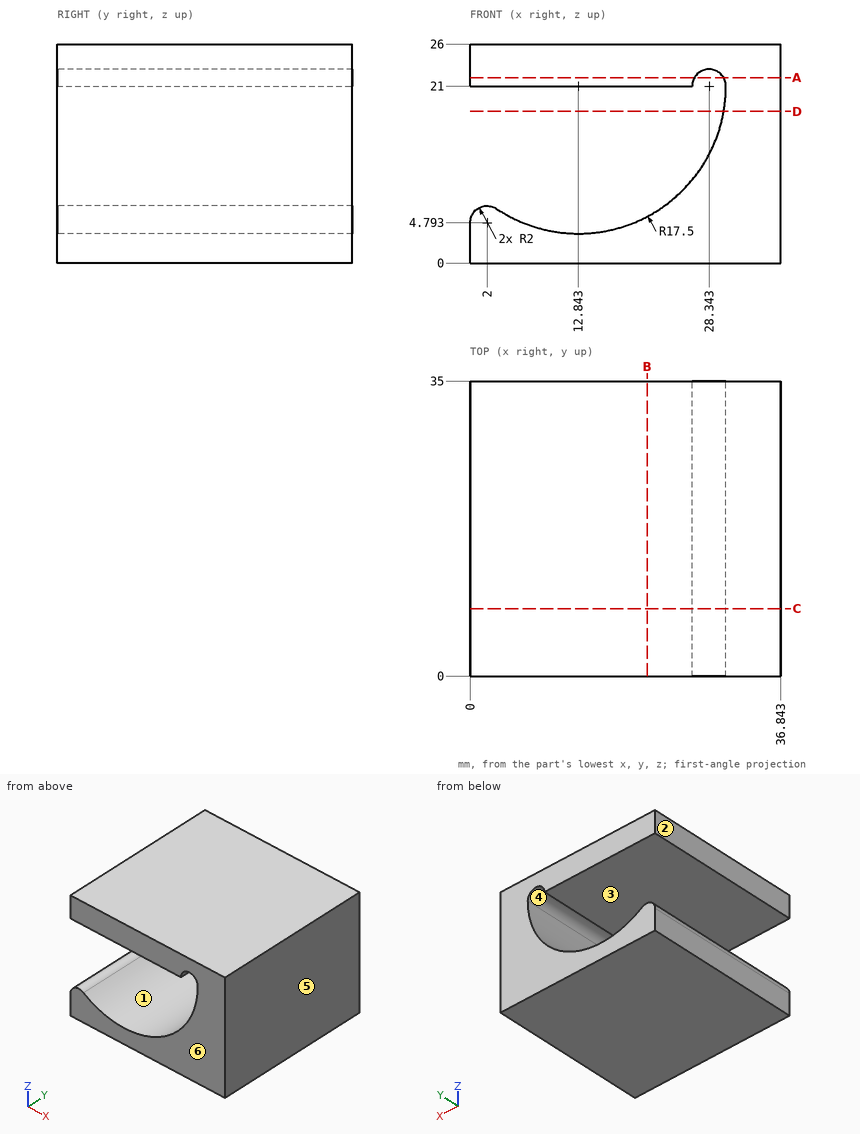
Part print with two shaded views. Sizes in mm from the minimum x, y, z corner. A direction names the side the tool comes from. Round coordinates to 2 decimals unless told otherwise and drop trailing zeros. Loops run counter-clockwise (first coordinate to the right, second up) from the corner with the lowest first, then second, coordinate; pieces in that order, holes last.
1. Slice it at A-A (z = 22). Give the cut face in (x, y) (1 decimal).
Solutions:
outline: (0, 0) - (26.6, 0) - (26.6, 35) - (0, 35) - close; (30.1, 0) - (36.8, 0) - (36.8, 35) - (30.1, 35) - close
2. Slice it at D-D (z = 18). Give the cut face in (x, y), and give its area (3 significant figures).
Solutions:
outline: (30.08, 0) - (36.84, 0) - (36.84, 35) - (30.08, 35) - close
area: 237 mm2
3. Two-plate mould, pull along X, no slides. Class the marked faces 4, 5 and 6: pulls with the +X half, pulls with the -X half, needs draft (parallel to the pull), parting line crosses it, or undercut.
Solutions:
face 4: undercut
face 5: pulls with the +X half
face 6: needs draft
4. 3-axis set-ups, long thin cutter, end or side, ignore diameter. For the marked faces 1, 2 and 3: which of +Z, -Z, +X, -X, +Y, -Y reach the whole face in a straight line?
Solutions:
face 1: +Y, -Y
face 2: +Z, -Z, -X, +Y, -Y
face 3: -X, +Y, -Y
5. Slice it at B-B (x = 21). Give the cut face in (y, z).
Solutions:
outline: (0, 0) - (35, 0) - (35, 5.52) - (0, 5.52) - close; (0, 21) - (35, 21) - (35, 26) - (0, 26) - close
6. Flat gauge pins, fed straight in: pin 1 (8 mm diameter, centred on x = 13, z = 16.5, fed in from +Y); pin 2 (6 mm diameter, centred on y = 13, z = 16.5, fed in from -X) (1 decimal). Where does each tip first touch, or does it go through?
Solutions:
pin 1: passes through
pin 2: stops at x = 28.7
7. Slice it at C-C (y = 8). Give the cut face in (x, z) (1 decimal).
Solutions:
outline: (0, 0) - (36.8, 0) - (36.8, 26) - (0, 26) - (0, 21) - (26.3, 21) arc R2 cw to (30.3, 21) arc R17.5 cw to (3.1, 6.5) arc R2 ccw to (0, 4.8) - close
8. Drill centre lines: line 1 along Z through (x, y) = (13, 17); line 2 along Z through (x, y) = (11, 2.5); line 3 along X through (y, z) = (27.5, 22.5) (1 decimal). Where is each one in solid material? Low to high.
Solutions:
line 1: z = 0 to 3.5, 21 to 26
line 2: z = 0 to 3.6, 21 to 26
line 3: x = 0 to 27, 29.7 to 36.8
